Here's how the part is built. I have some questions about the finished solid (model axes, mm). A direction names the side the tool comes from. Coordinates: 2 decimals unless noted, no trailing zeros. Write each loop counter-clockwise with the first axis right and the second up, starting at its lowest first coordinate (ties: lowest second). Pieces come first, ordered by that corner, then holes. Notation, with made-up numbers: (55.25, 33) -> (87.25, 33) arc R14 ccw to (87.25, 57) -> close; hole circle Ø9 at (50.5, -3.5). An arc over 180 degrees is marked (long way). Use a Markdown table: item, result. Add a question column.
```python
from build123d import *

# Parameters (mm, degrees)
SCALE1_SCALE = 0.6


with BuildPart() as part:
    # Sketch1 → Revolve1 (revolve)
    with BuildSketch(Plane(origin=(0, 0, 0), x_dir=(0, 0, -1), z_dir=(1, 0, 0))):
        Polygon((16.7, 3.5), (20.7, 3.5), (20.7, 4.5), (-20.7, 4.5), (-20.7, 3.5), (-16.7, 3.5), (-16.7, 2), (16.7, 2), align=None)
    revolve(axis=Axis((0, 0, 16.930047934), (0, 0, -1)))


with BuildPart() as part_1:
    # Scale1: scaled about (0, 0, 0)
    add(part.part.scale(SCALE1_SCALE))


solid = part_1.part
```
Q1. Suppose I cut it at C-C, the plane z = -7.25. Write out the boundary of the cut face in (x, y).
Q2. Will these pins go through, and if not, where does the flat tip stop? pin 1 (1 mm diameter, centred on x = 2, z = -5.5, fed in from +Y) (3 decimals); pin 2 (2 mm diameter, centred on x = -2, z = -2.5, fed in from -Y); pin 3 (1 mm diameter, centred on y = 1, z = 9, fed in from +X).
Q3. Which directions (+Z, -Z, +X, -X, +Y, -Y) give clear straight access to the entire face, cutting with the end or side of a thin tool? Please do faces 1 (the flat face through (-1, -1, -10.02)), 2 (the flat face through (-1, 1, 10.02)), 3 (the cylindrical face through (1.01, 0.65, -0.14)).
Q4. Suppose I cut it at A-A, the plane y = 0. Write out the boundary of the cut face in (x, z), and give its area (3 significant figures).
Q5. Suppose I cut it at D-D, the plane x = 1.8. Write out the boundary of the cut face in (y, z), and give its area (3 significant figures).
Q6. Please list where these lines run through material, in increasing order: line 1 (X direction, y = 0, z = 11.1); line 2 (X direction, y = 0, z = 3.75); line 3 (Z direction, x = 1.8, y = 0.8).
Q7. Thinking about a two-plate mould opening in Y: for faces 4 (the cylindrical face through (0.631, 2.003, -11.237)), 5 (the cylindrical face through (0.811, 2.575, 0.174)), which applies, released by +Y, released by -Y, zero draft, split by the parting line, or undercut?
Answer key:
| question | item | result |
|---|---|---|
| 1 | outline | circle Ø5.4 at (0, 0); hole circle Ø2.4 at (0, 0) |
| 2 | pin 1 | stops at y = 2.245 |
| 2 | pin 2 | stops at y = -2.51 |
| 2 | pin 3 | stops at x = 2.65 |
| 3 | face 1 | -Z |
| 3 | face 2 | +Z |
| 3 | face 3 | +Z, -Z |
| 4 | outline | (-2.7, -12.42) -> (-2.1, -12.42) -> (-2.1, -10.02) -> (-1.2, -10.02) -> (-1.2, 10.02) -> (-2.1, 10.02) -> (-2.1, 12.42) -> (-2.7, 12.42) -> close; (1.2, -10.02) -> (2.1, -10.02) -> (2.1, -12.42) -> (2.7, -12.42) -> (2.7, 12.42) -> (2.1, 12.42) -> (2.1, 10.02) -> (1.2, 10.02) -> close |
| 4 | area | 65.9 mm^2 |
| 5 | outline | (-2.01, -12.42) -> (-1.08, -12.42) -> (-1.08, -10.02) -> (1.08, -10.02) -> (1.08, -12.42) -> (2.01, -12.42) -> (2.01, 12.42) -> (1.08, 12.42) -> (1.08, 10.02) -> (-1.08, 10.02) -> (-1.08, 12.42) -> (-2.01, 12.42) -> close |
| 5 | area | 89.6 mm^2 |
| 6 | line 1 | x = -2.7 to -2.1, 2.1 to 2.7 |
| 6 | line 2 | x = -2.7 to -1.2, 1.2 to 2.7 |
| 6 | line 3 | z = -10.02 to 10.02 |
| 7 | face 4 | undercut |
| 7 | face 5 | split by the parting line |
